Work out the finished part from the listing and answer in its coordinate system (mm). Face numbers are marked on the shaded views. A direction names the side the tool comes from. Coordinates: 2 decimals unless noted, no trailing zeros. Order: outer loops, then holes, each group sorted by start corner. A loop starts at its lowest first (then second) coordinate and runs counter-clockwise, first axis right, second up.
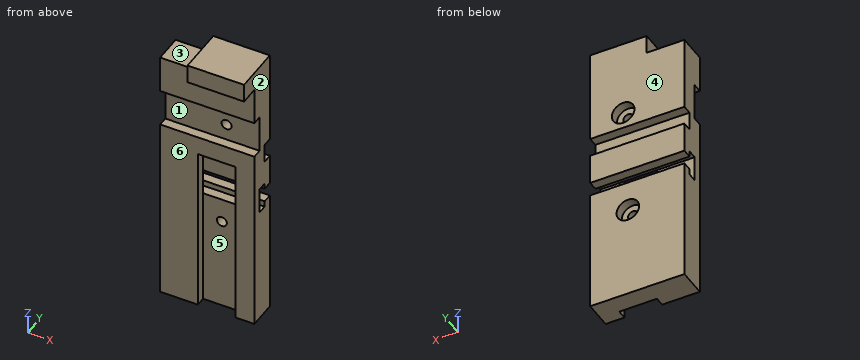
Autodesk Inventor part; units mm, degrees
ref_plane "YZ Plane" through (0, 0, 0) normal (1, 0, 0) x (0, 1, 0)
ref_plane "XZ Plane" through (0, 0, 0) normal (0, 1, 0) x (-1, 0, 0)
sketch "Sketch3" plane through (0, 0, 0) normal (0, 0, 1) x (1, 0, 0)
  line L0 (0, -9.525) -> (9.525, -9.525)
  line L1 (9.525, -9.525) -> (9.525, 0)
  line L2 (0, 0) -> (0, -9.525) construction
  line L3 (0, 0) -> (9.525, 0) construction
  line L4 (0, -9.525) -> (-9.525, -9.525)
  line L5 (-9.525, -9.525) -> (-9.525, 0)
  line L6 (9.525, 0) -> (73.025, 0)
  line L7 (-187.325, 0) -> (-187.325, 19.05)
  line L8 (-187.325, 0) -> (-9.525, 0)
  line L9 (73.025, 0) -> (73.025, 19.05)
  line L10 (73.025, 19.05) -> (-187.325, 19.05)
  dimension "d0" = 9.525
  dimension "d1" = 9.525
  dimension "d6" = 63.5
  dimension "d8" = 19.05
  dimension "d9" = 177.8
extrude "Extrusion1" add sketch "Sketch3" along normal mid plane 355.6
sketch "Sketch4" plane through (0, 0, 177.8) normal (0, 0, 1) x (1, 0, 0)
  line L0 (-187.325, 19.05) -> (73.025, 19.05) construction
  line L1 (0, 19.05) -> (0, -9.525) construction
  line L2 (9.525, -9.525) -> (-9.525, -9.525) construction
  line L3 (0, -9.525) -> (-22.225, -9.525)
  line L4 (-22.225, -9.525) -> (-22.225, 19.05)
  line L5 (-22.225, 19.05) -> (0, 19.05)
  line L6 (187.325, 19.05) -> (-73.025, 19.05) construction
  line L7 (0, -9.525) -> (22.225, -9.525)
  line L8 (22.225, -9.525) -> (22.225, 19.05)
  line L9 (0, 19.05) -> (22.225, 19.05)
  point P0 (0, 0)
  dimension "d12" = 22.225
extrude "Extrusion2" add sketch "Sketch4" along normal blind 12.7
mirror "Mirror1" about plane through (0, 0, 0) normal (0, 0, 1) of "Extrusion2"
sketch "Sketch6" plane through (-187.325, 0, -177.8) normal (0, -1, 0) x (1, 0, 0)
  line L0 (82.55, 165.1) -> (88.9, 165.1)
  line L1 (88.9, 165.1) -> (88.9, 190.5)
  line L2 (88.9, 190.5) -> (82.55, 190.5)
  line L3 (82.55, 190.5) -> (82.55, 165.1)
  line L4 (82.55, 165.1) -> (88.9, 190.5) construction
  line L5 (88.9, 165.1) -> (82.55, 190.5) construction
  line L6 (177.8, 0) -> (177.8, 355.6)
  point P0 (187.325, 177.8)
  point P1 (85.725, 177.8)
  dimension "d16" = 12.7
  dimension "d18" = 6.35
  dimension "d19" = 88.9
extrude "Extrusion3" cut sketch "Sketch6" against normal through all
sketch "Sketch7" plane through (0, 0, 177.8) normal (0, 0, 1) x (1, 0, 0)
  line L0 (-187.325, 19.05) -> (-22.225, 19.05)
  line L1 (-161.925, 19.05) -> (-117.475, 19.05)
  line L2 (-117.475, 19.05) -> (-117.475, -12.7)
  line L3 (-117.475, -12.7) -> (-161.925, -12.7)
  line L4 (-161.925, -12.7) -> (-161.925, 19.05)
  line L5 (-187.325, 19.05) -> (-187.325, 0)
  point P0 (0, 0)
  dimension "d22" = 44.45
  dimension "d23" = 31.75
  dimension "d24" = 25.4
extrude "Extrusion4" add sketch "Sketch7" along normal blind 12.7
mirror "Mirror2" about plane through (0, 0, 0) normal (0, 0, 1) of "Extrusion4"
sketch "Sketch9" plane through (73.025, 0, 177.8) normal (1, 0, 0) x (0, 0, -1)
  line L0 (355.6, 19.05) -> (0, 19.05)
  line L1 (50.8, 19.05) -> (63.5, 19.05)
  line L2 (63.5, 19.05) -> (63.5, 12.7)
  line L3 (63.5, 12.7) -> (50.8, 12.7)
  line L4 (50.8, 12.7) -> (50.8, 19.05)
  line L5 (0, 0) -> (0, 19.05)
  point P0 (177.8, 0)
  dimension "d28" = 12.7
  dimension "d29" = 6.35
  dimension "d30" = 50.8
extrude "Extrusion5" cut sketch "Sketch9" against normal through all
mirror "Mirror3" about plane through (0, 0, 0) normal (0, 0, 1) of "Extrusion5"
sketch "Sketch12" plane through (73.025, 0, 177.8) normal (1, 0, 0) x (0, 0, -1)
  line L0 (355.6, 0) -> (0, 0) construction
  line L1 (88.9, 0) -> (88.9, 16.5009) construction
  line L2 (0, 0) -> (0, 19.05)
  line L3 (50.8, 19.05) -> (0, 19.05)
  line L4 (84.1375, 19.05) -> (84.1375, 12.7)
  line L5 (84.1375, 12.7) -> (80.1624, 12.7)
  line L6 (80.1624, 12.7) -> (80.1624, 6.35)
  line L7 (80.1624, 6.35) -> (88.9, 6.35)
  line L8 (93.6625, 19.05) -> (93.6625, 12.7)
  line L9 (93.6625, 12.7) -> (97.6376, 12.7)
  line L10 (97.6376, 12.7) -> (97.6376, 6.35)
  line L11 (97.6376, 6.35) -> (88.9, 6.35)
  line L12 (84.1375, 19.05) -> (93.6625, 19.05)
  point P0 (177.8, 0)
  dimension "d46" = 88.9
  dimension "d47" = 4.7625
  dimension "d48" = 6.35
  dimension "d49" = 6.35
  dimension "d50" = 8.7376
extrude "Extrusion8" cut sketch "Sketch12" against normal through all
mirror "Mirror4" about plane through (0, 0, 0) normal (0, 0, 1) of "Extrusion8"
ref_plane "Work Plane1" through (-57.15, 0, 177.8) normal (1, 0, 0) x (0, 0, -1)
sketch "Sketch13" plane through (-57.15, 0, 177.8) normal (1, 0, 0) x (0, 0, -1)
  line L0 (25.4, 0) -> (50.8, 0)
  line L1 (50.8, 0) -> (50.8, 6.35)
  line L2 (50.8, 6.35) -> (25.4, 6.35)
  line L3 (25.4, 6.35) -> (25.4, 0)
  line L4 (0, 0) -> (0, 19.05)
  point P0 (177.8, 0)
  dimension "d54" = 25.4
  dimension "d55" = 6.35
  dimension "d56" = 25.4
extrude "Extrusion9" cut sketch "Sketch13" along normal mid plane 260.35
mirror "Mirror5" about plane through (0, 0, 0) normal (0, 0, 1) of "Extrusion9"
sketch "Sketch14" plane through (0, 0, 0) normal (0, 0, 1) x (1, 0, 0)
  line L0 (-187.325, 0) -> (-161.925, 0)
  line L1 (-161.925, 0) -> (-136.525, 0)
  line L2 (-136.525, 0) -> (-136.525, 6.35)
  line L3 (-136.525, 6.35) -> (-161.925, 6.35)
  line L4 (-161.925, 6.35) -> (-161.925, 0)
  line L5 (-187.325, 19.05) -> (-187.325, 0)
  point P0 (0, 0)
  dimension "d59" = 25.4
  dimension "d60" = 6.35
  dimension "d61" = 25.4
extrude "Extrusion10" cut sketch "Sketch14" along normal mid plane 228.6
mirror "Mirror6" about plane through (-57.15, 0, 177.8) normal (1, 0, 0) of "Extrusion10"
sketch "Sketch16" plane through (-161.925, 6.35, -80.1624) normal (0, -1, 0) x (1, 0, 0)
  circle A0 centre (12.7, 143.6624) radius 3.3782
  line L0 (0, 194.4624) -> (25.4, 194.4624)
  line L1 (0, -34.1376) -> (0, 194.4624)
  point P0 (161.925, 80.1624)
  dimension "d71" = 6.7564
  dimension "d72" = 50.8
  dimension "d73" = 12.7
extrude "Extrusion11" cut sketch "Sketch16" against normal through all
sketch "Sketch17" plane through (-187.325, 19.05, 84.1375) normal (0, 1, 0) x (1, 0, 0)
  circle A0 centre (38.1, 20.6375) radius 3.3782
  circle A1 centre (38.1, 20.6375) radius 7.62
  point P0 (187.325, 84.1375)
  dimension "d76" = 15.24
extrude "Extrusion12" cut sketch "Sketch17" against normal blind 6.35
mirror "Mirror7" about plane through (0, 0, 0) normal (0, 0, 1) of "Extrusion12", "Extrusion11"
mirror "Mirror8" about plane through (-57.15, 0, 177.8) normal (1, 0, 0) of "Extrusion12", "Extrusion11", "Mirror7"
sketch "Sketch18" plane through (-171.45, 6.35, 152.4) normal (0, -1, 0) x (1, 0, 0)
  circle A0 centre (203.2, -14.094) radius 3.3782
  line L0 (228.6, 0) -> (228.6, -25.4)
  point P0 (171.45, -152.4)
  dimension "d79" = 6.7564
  dimension "d80" = 25.4
extrude "Extrusion13" cut sketch "Sketch18" against normal through all
sketch "Sketch19" plane through (22.225, 19.05, 177.8) normal (0, 1, 0) x (1, 0, 0)
  circle A0 centre (9.525, 39.494) radius 3.3782
  circle A1 centre (9.525, 39.494) radius 7.62
  point P0 (-22.225, 177.8)
  dimension "d83" = 15.24
extrude "Extrusion14" cut sketch "Sketch19" against normal blind 6.35
mirror "Mirror9" about plane through (-57.15, 0, 177.8) normal (1, 0, 0) of "Extrusion13", "Extrusion14"
mirror "Mirror10" about plane through (0, 0, 0) normal (0, 0, 1) of "Extrusion14", "Extrusion13", "Mirror9"
split "Split3" plane through (-57.15, 0, 177.8) removes the side toward (1, 0, 0)
split "Split4" plane through (0, 0, 0) removes the side toward (0, 0, -1)
ref_plane "Work Plane2" through (-123.825, 0, 177.8) normal (1, 0, 0) x (0, 0, -1)
split "Split5" plane through (-123.825, 0, 177.8) removes the side toward (1, 0, 0)
equation "\"d10\" = length"
equation "\"width\" = 260.35"
equation "\"length\" = 355.6"
equation "\"d53\" = -0.5 * width"
properties part number "BandSawJigBottomA" material "LCP Plastic"
1. The part is cut by section B-B (y = 16). Count the separate pieces of the cut face and the enclosed holes in it, plus the area to 4 significant figures.
2. The mould has two halves that part along Z. Classify the marked faces 1, 2 and 3: released by +Z, released by -Z, zero draft, split by the parting line, or undercut.
3. The part is cut by section A-A (z = 63.5). Determine the outline of the cut face in (x, y) (3 decimals).
4. Flat-ended cylindrical pins translate along their axes: pin 1 (4.5 mm diameter, centred on x = -168, z = 96.5, fed in from -Y); pin 2 (9 mm diameter, centred on x = -146.05, z = 138.306, fed in from -Y); pin 3 (4 mm diameter, centred on x = -133, z = 87.5, fed in from +Y). Find the tip coordinate at first contact, or state that the pin passes through.
5. The part is cut by section D-D (z = 149). Determine the outline of the cut face in (x, y) (3 decimals).
6. For the marked faces 4, 5 and 6, determine the directions among +Z, -Z, +X, -X, +Y, -Y from which every point of the face is accessible in a straight line to the end or side of a thin tool.
7. Consider probe 1 along X at (y, z) = (3, 32.5) (3 decimals); probe 2 along Z at (x, y) = (-180, 6); probe 3 along Z at (x, y) = (-146.05, 15). Determine where each line is inside the solid, lowest interval first.
8. The part is cut by section C-C (x = -180.5). Determine the outline of the cut face in (y, z), plus the area to 3 significant figures.
Worked out:
1. separate pieces: 3
1. enclosed holes: 2
1. area: 10,000 mm2
2. face 1: undercut
2. face 2: zero draft
2. face 3: released by +Z
3. outline: (-187.325, 0) - (-161.925, 0) - (-161.925, 6.35) - (-152.603, 6.35) - (-152.603, 12.7) - (-156.845, 12.7) - (-156.845, 19.05) - (-187.325, 19.05) - close; (-145.847, 6.35) - (-136.525, 6.35) - (-136.525, 0) - (-123.825, 0) - (-123.825, 19.05) - (-141.605, 19.05) - (-141.605, 12.7) - (-145.847, 12.7) - close
4. pin 1: stops at y = 0
4. pin 2: stops at y = 6.35
4. pin 3: stops at y = 6.35
5. outline: (-187.325, 6.35) - (-123.825, 6.35) - (-123.825, 19.05) - (-187.325, 19.05) - close
6. face 4: +Z, -Z, +X, -X, +Y
6. face 5: -Z, -Y
6. face 6: -Z, +X, -X, -Y
7. probe 1: x = -187.325 to -161.925, -136.525 to -123.825
7. probe 2: z = 0 to 127, 152.4 to 177.8
7. probe 3: z = 0 to 56.57, 70.43 to 84.14, 93.66 to 114.3, 127 to 130.69, 145.93 to 190.5
8. outline: (0, 0) - (19.05, 0) - (19.05, 84.14) - (12.7, 84.14) - (12.7, 80.16) - (6.35, 80.16) - (6.35, 97.64) - (12.7, 97.64) - (12.7, 93.66) - (19.05, 93.66) - (19.05, 114.3) - (12.7, 114.3) - (12.7, 127) - (19.05, 127) - (19.05, 177.8) - (0, 177.8) - (0, 152.4) - (6.35, 152.4) - (6.35, 127) - (0, 127) - close
8. area: 2,970 mm2
